Source: three-view drawing plus pictorial views. Frame: mm from the lowest corner of the part. Coordinates: 2 decimals unless noted, no trailing zeros. Write each loop counter-clockwise with the first axis right and the second up, starting at its lowest first coordinate (ties: lowest second). Pieces come first, ordered by that corner, then holes. Notation, with made-up numbers: (-31.5, -38.5) -> (-4.5, -38.5) arc R36 cw to (-4.5, -3.5) -> close; hole circle Ø10 at (52.25, -5). An arc over 180 degrees is marked (long way). One line per question, with ' | ' between items. Start each with the question number.
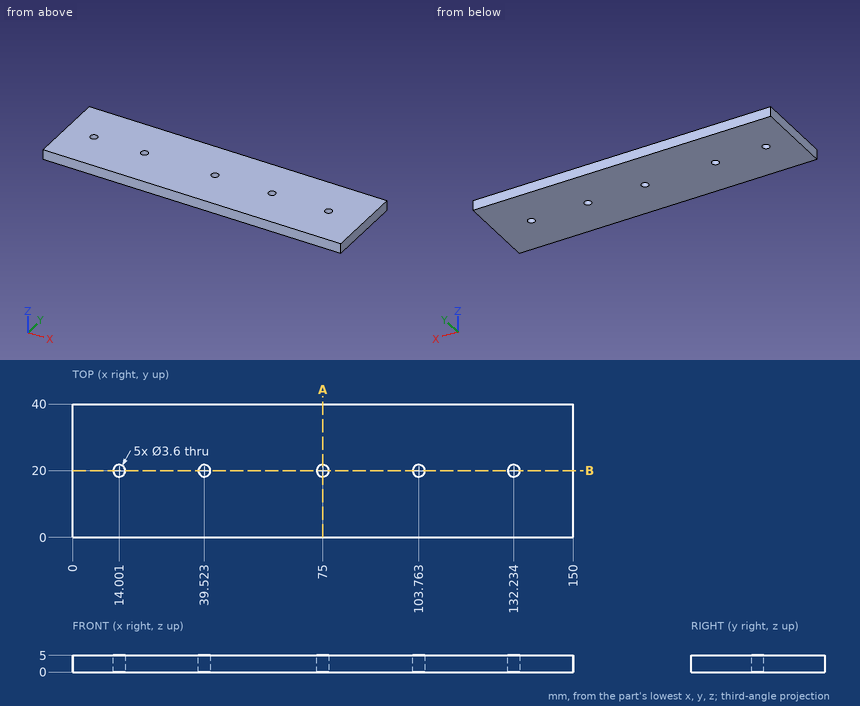
1) Section B-B, the plane y = 20. Return loops of the section in (x, z) (1 decimal).
2) Ray query, line 1 (Y direction, x = 75, z = 2.6); line 2 (X direction, y = 18.5, z = 1.75) (1 decimal); line 3 (X direction, y = 19.5, z = 3.55) (1 decimal). Return the intervals inside material, ascending.
3) Section A-A, the plane x = 75. Return loops of the section in (y, z), then the cut area to 3 significant figures.
4) First-contact query: P1, Ø4, axis at x = 132.23, y = 20, coming from the -Z side. Flat tip, straight axial feed; report the tip coordinate or a pass-through.
Answer block:
1) outline: (0, 0) -> (12.2, 0) -> (12.2, 5) -> (0, 5) -> close; (15.8, 0) -> (37.7, 0) -> (37.7, 5) -> (15.8, 5) -> close; (41.3, 0) -> (73.2, 0) -> (73.2, 5) -> (41.3, 5) -> close; (76.8, 0) -> (102, 0) -> (102, 5) -> (76.8, 5) -> close; (105.6, 0) -> (130.4, 0) -> (130.4, 5) -> (105.6, 5) -> close; (134, 0) -> (150, 0) -> (150, 5) -> (134, 5) -> close
2) line 1: y = 0 to 18.2, 21.8 to 40 | line 2: x = 0 to 13, 15 to 38.5, 40.5 to 74, 76 to 102.8, 104.8 to 131.2, 133.2 to 150 | line 3: x = 0 to 12.3, 15.7 to 37.8, 41.3 to 73.3, 76.7 to 102, 105.5 to 130.5, 134 to 150
3) outline: (0, 0) -> (18.2, 0) -> (18.2, 5) -> (0, 5) -> close; (21.8, 0) -> (40, 0) -> (40, 5) -> (21.8, 5) -> close | area: 182 mm2
4) P1: stops at z = 0
